```python
from build123d import *

# Parameters (mm, degrees)
SKETCH_R  = 2.1
PAD_DEPTH = 1


with BuildPart() as part:
    # Sketch → Pad (new body)
    with BuildSketch(Plane.XY):
        with BuildLine():
            Line((-3.5, 15), (43.5, 15))
            ThreePointArc((45, 13.5), (44.56066, 14.56066), (43.5, 15))
            Line((45, 13.5), (45, -3.5))
            ThreePointArc((43.5, -5), (44.56066, -4.56066), (45, -3.5))
            Line((43.5, -5), (-3.5, -5))
            ThreePointArc((-5, -3.5), (-4.56066, -4.56066), (-3.5, -5))
            Line((-5, -3.5), (-5, 13.5))
            ThreePointArc((-3.5, 15), (-4.56066, 14.56066), (-5, 13.5))
        make_face()
        Circle(SKETCH_R, mode=Mode.SUBTRACT)
        with Locations((0, 10)):
            Circle(SKETCH_R, mode=Mode.SUBTRACT)
        with Locations((10, 0)):
            Circle(SKETCH_R, mode=Mode.SUBTRACT)
        with Locations((20, 0)):
            Circle(SKETCH_R, mode=Mode.SUBTRACT)
        with Locations((30, 0)):
            Circle(SKETCH_R, mode=Mode.SUBTRACT)
        with Locations((40, 0)):
            Circle(SKETCH_R, mode=Mode.SUBTRACT)
        with Locations((10, 10)):
            Circle(SKETCH_R, mode=Mode.SUBTRACT)
        with Locations((20, 10)):
            Circle(SKETCH_R, mode=Mode.SUBTRACT)
        with Locations((30, 10)):
            Circle(SKETCH_R, mode=Mode.SUBTRACT)
        with Locations((40, 10)):
            Circle(SKETCH_R, mode=Mode.SUBTRACT)
    extrude(amount=PAD_DEPTH)


solid = part.part
```
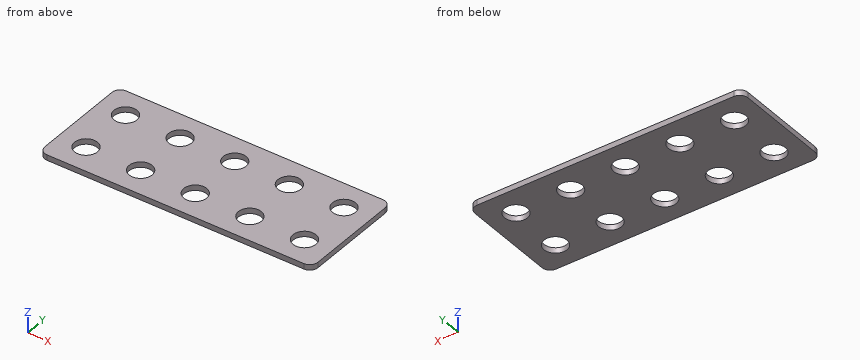
CAD build for the part. Positions are in the model's coordinates, mm. Round coordinates to 2 decimals unless told otherwise and drop trailing zeros. Order: outer loops, then holes, each group sorted by start corner. A loop starts at its lowest first (then second) coordinate and runs counter-clockwise, first axis right, second up.
Item 1: Saw through at B-B on x = 0. Write the cut outline in (y, z).
Item 2: Pin check, flat tip, straight feed: pin 1 (6.5 mm diameter, centred on x = 10, y = 10, fed in from +Z). Stop position of the tip, or through.
Item 3: Saw through at C-C on y = 10. Write the cut outline in (x, z).
Item 4: Probe line 1 along Y through (x, z) = (0, 0.4); line 2 along Y through (x, z) = (19, 0.9); line 3 along X through (y, z) = (-0.5, 0.5). List the from-to ranges inside material, lowest first.
Item 5: Saw through at A-A on z = 0.65. State how many separate pieces and enclosed holes the cut face has, then the cut area to 3 significant figures.
Reported:
1. outline: (-5, 0) - (-2.1, 0) - (-2.1, 1) - (-5, 1) - close; (2.1, 0) - (7.9, 0) - (7.9, 1) - (2.1, 1) - close; (12.1, 0) - (15, 0) - (15, 1) - (12.1, 1) - close
2. pin 1: stops at z = 1
3. outline: (-5, 0) - (-2.1, 0) - (-2.1, 1) - (-5, 1) - close; (2.1, 0) - (7.9, 0) - (7.9, 1) - (2.1, 1) - close; (12.1, 0) - (17.9, 0) - (17.9, 1) - (12.1, 1) - close; (22.1, 0) - (27.9, 0) - (27.9, 1) - (22.1, 1) - close; (32.1, 0) - (37.9, 0) - (37.9, 1) - (32.1, 1) - close; (42.1, 0) - (45, 0) - (45, 1) - (42.1, 1) - close
4. line 1: y = -5 to -2.1, 2.1 to 7.9, 12.1 to 15
4. line 2: y = -5 to -1.85, 1.85 to 8.15, 11.85 to 15
4. line 3: x = -5 to -2.04, 2.04 to 7.96, 12.04 to 17.96, 22.04 to 27.96, 32.04 to 37.96, 42.04 to 45
5. separate pieces: 1
5. enclosed holes: 10
5. area: 860 mm2
